Part model, mm, in its own coordinate system. A direction names the side the tool comes from. Coordinates: 2 decimals unless noted, no trailing zeros. Loops run counter-clockwise (first coordinate to the right, second up) from the corner with the lowest first, then second, coordinate; pieces in that order, holes last. Notation, with made-up numbers: M -3,70 L 41,70 A30 cw 41,93 Z; hole C 60,-5 d2. An arc over 180 degrees is marked long. Answer as CSV lines item,"result". Start each with the question number.
from build123d import *

# Parameters (mm, degrees)
F0_W      = 406.4
F0_H      = 1143
F1_DEPTH  = 812.8
F2_W      = 25.4
F2_H      = 1143
F3_DEPTH  = 25.4
F4_W      = 508
F4_H      = 194.733333
F4_H_2    = 194.733334
F5_DEPTH  = 12.7
F6_DEPTH  = 406.401
F7_W      = 170.104802
F7_H      = 44.162155
F8_DEPTH  = 12.7
F9_W      = 203.2
F9_H      = 939.8
F10_DEPTH = 693.42


with BuildPart() as f1:
    # F0 (on Top) → F1 (new body)
    with BuildSketch(Plane.XY):
        Rectangle(F0_W, F0_H)
    extrude(amount=F1_DEPTH)

    # F2 (on face) → F3 (join)
    with BuildSketch(Plane.XY.offset(812.8)):
        with Locations((215.9, 0)):
            Rectangle(F2_W, F2_H)
    extrude(amount=-F3_DEPTH)

    # F4 (on face) → F5 (join)
    with BuildSketch(Plane.YZ.offset(203.2)):
        with Locations((-266.7, 664.633333)):
            Rectangle(F4_W, F4_H)
        with Locations((266.7, 664.633333)):
            Rectangle(F4_W, F4_H)
        with Locations((266.7, 444.5)):
            Rectangle(F4_W, F4_H_2)
        with Locations((-266.7, 444.5)):
            Rectangle(F4_W, F4_H_2)
        with Locations((-266.7, 224.366666)):
            Rectangle(F4_W, F4_H)
        with Locations((266.7, 224.366666)):
            Rectangle(F4_W, F4_H)
    extrude(amount=F5_DEPTH)

    # F4 (on face) → F6 (cut, through all)
    with BuildSketch(Plane.YZ.offset(203.2)):
        with BuildLine():
            Line((342.9, 76.2), (-342.9, 76.2))
            ThreePointArc((-342.9, 76.2), (-396.781537, 53.881537), (-419.1, 0))
            Line((-419.1, 0), (419.1, 0))
            ThreePointArc((419.1, 0), (396.781537, 53.881537), (342.9, 76.2))
        make_face()
    extrude(amount=-F6_DEPTH, mode=Mode.SUBTRACT)

    # F7 (on face) → F8 (join)
    with BuildSketch(Plane.YZ.offset(215.9)):
        with Locations((-266.7, 664.633333)):
            Rectangle(F7_W, F7_H)
        with Locations((266.7, 664.633333)):
            Rectangle(F7_W, F7_H)
        with Locations((266.7, 444.262933)):
            Rectangle(F7_W, F7_H)
        with Locations((266.7, 223.892533)):
            Rectangle(F7_W, F7_H)
        with Locations((-266.7, 223.892533)):
            Rectangle(F7_W, F7_H)
        with Locations((-266.7, 444.262933)):
            Rectangle(F7_W, F7_H)
    extrude(amount=F8_DEPTH)

    # F9 (on face) → F10 (cut)
    with BuildSketch(Plane(origin=(0, 0, 0), x_dir=(1, 0, 0), z_dir=(0, 0, -1))):
        Rectangle(F9_W, F9_H)
    extrude(amount=-F10_DEPTH, mode=Mode.SUBTRACT)


solid = f1.part
Q1. Wall check: L1, parallel to Y at x = -42.5, z = 535; L2, parallel to X at y = 201, z = 677.5; L3, parallel to X at y = 71, z = 644. Give the ranges that are in metal, low to high.
Q2. Two-plate mould, pull along Z, no slides. Class faces 1 (the face through (153, 5, 76.2)), 2 (the face through (228.6, -268, 445)), 3 (the face through (215.9, 263, 688)): +Z half, -Z half, draft (parallel to the pull), parting line (faces both ways), or undercut.
Q3. Flat gauge pins, fed straight in: P1, Ø3, axis at y = -44, z = 413, coming from the +X side; P2, Ø10, axis at x = 208.5, z = 712, coming from the -Y side; P3, Ø10, axis at x = 206.5, y = 175.5, coming from the -Z side. Where does each tip first touch, or does it go through?
Q4. Slice it at D-D, the plane z = 99. Write the cut outline in (x, y), and give its area (3 significant figures).
Q5. Tool access for faces 4 (the face through (-101.6, 7, 342)), 5 (the face through (-151.689, -396.186, 54.471)), 6 (the face through (10, -571.5, 412)): list every direction of +Z, -Z, +X, -X, +Y, -Y with a clear straight run to the whole face (end or side of a thin tool).
Q6. Slice it at A-A, the plane z = 590. Write the cut outline in (x, y), and give its area (3 significant figures).
Q7. Slice it at B-B, the plane x = -129.5. Write the cut outline in (y, z).
Solved:
1,L1,"y = -571.5 to -469.9, 469.9 to 571.5"
1,L2,"x = -203.2 to -101.6, 101.6 to 228.6"
1,L3,"x = -203.2 to -101.6, 101.6 to 215.9"
2,face 1,"-Z half"
2,face 2,"draft"
2,face 3,"undercut"
3,P1,"stops at x = 215.9"
3,P2,"stops at y = -520.7"
3,P3,"stops at z = 76.2"
4,outline,"M -203.2,-571.5 L 203.2,-571.5 L 203.2,571.5 L -203.2,571.5 Z; hole M -101.6,-469.9 L 101.6,-469.9 L 101.6,469.9 L -101.6,469.9 Z"
4,area,"274,000 mm2"
5,face 4,"-Z"
5,face 5,"-Z, +X, -X"
5,face 6,"+Z, -Z, +X, -X, -Y"
6,outline,"M -203.2,-571.5 L 203.2,-571.5 L 203.2,-520.7 L 215.9,-520.7 L 215.9,-12.7 L 203.2,-12.7 L 203.2,12.7 L 215.9,12.7 L 215.9,520.7 L 203.2,520.7 L 203.2,571.5 L -203.2,571.5 Z; hole M -101.6,-469.9 L 101.6,-469.9 L 101.6,469.9 L -101.6,469.9 Z"
6,area,"286,000 mm2"
7,outline,"M -571.5,0 L -419.1,0 A76.2 cw -342.9,76.2 L 342.9,76.2 A76.2 cw 419.1,0 L 571.5,0 L 571.5,812.8 L -571.5,812.8 Z"
